Part model, mm, in its own coordinate system. Round coordinates to 2 decimals unless told otherwise and drop trailing zeros. Loops run counter-clockwise (first coordinate to the right, second up) from the corner with the lowest first, then second, coordinate; pieces in that order, holes last.
1) Band-saw the part on D-D, the plane x = 21.5. Write the cut outline in (y, z), then the cut area to 3 significant figures.
2) Band-saw the part on A-A, the plane y = -45. Write the cut outline in (x, z), then the cut area to 3 significant figures.
3) Mould opens along Y. For faces 1 (the flat face through (-1, 1, 2)), 2 (the cylindrical face through (-18, 0, 1)), 3 (the cylindrical face through (23.48, -49.39, 0.99)) say: +Y half, -Y half, draft (parallel to the pull), parting line (faces both ways), or undercut.
4) Band-saw the part on B-B, the plane x = -22.5. Write the cut outline in (y, z), then the cut area to 3 significant figures.
5) Probe line 1 (Y direction, x = -22.5, z = 1.2); line 2 (X direction, y = -41, z = 1.6); line 3 (X direction, y = 47, z = 0.55). List the from-to ranges inside material, lowest first.
6) Band-saw the part on C-C, the plane z = 1.4. Write the cut outline in (x, y).
from build123d import *

# Parameters (mm, degrees)
SKETCH_1_W        = 90
SKETCH_1_H        = 135
EXTRUDE_1_DEPTH   = 2
CHAMFER_1_SIZE    = 2
HOLE_WIZARD_M81_D = 9


with BuildPart() as part:
    # Эскиз1 → Бобышка-Вытянуть1 (new body)
    with BuildSketch(Plane.XY):
        Rectangle(SKETCH_1_W, SKETCH_1_H)
    extrude(amount=EXTRUDE_1_DEPTH)

    # Фаска1
    chamfer_1_edges = [part.edges().sort_by_distance(p)[0] for p in [
        (45, -67.5, 1),
        (-45, -67.5, 1),
        (-45, 67.5, 1),
        (45, 67.5, 1),
    ]]
    chamfer(chamfer_1_edges, length=CHAMFER_1_SIZE)

    # Отверстие с зазором M81 (through all)
    with Locations(Plane.XY.offset(2)):
        with Locations((-22.5, 45), (22.5, 45), (22.5, 0), (-22.5, 0), (-22.5, -45), (22.5, -45)):
            Hole(HOLE_WIZARD_M81_D / 2)


solid = part.part
Reported:
1. outline: (-67.5, 0) - (-49.39, 0) - (-49.39, 2) - (-67.5, 2) - close; (-40.61, 0) - (-4.39, 0) - (-4.39, 2) - (-40.61, 2) - close; (4.39, 0) - (40.61, 0) - (40.61, 2) - (4.39, 2) - close; (49.39, 0) - (67.5, 0) - (67.5, 2) - (49.39, 2) - close
1. area: 217 mm2
2. outline: (-45, 0) - (-27, 0) - (-27, 2) - (-45, 2) - close; (-18, 0) - (18, 0) - (18, 2) - (-18, 2) - close; (27, 0) - (45, 0) - (45, 2) - (27, 2) - close
2. area: 144 mm2
3. face 1: draft
3. face 2: undercut
3. face 3: undercut
4. outline: (-67.5, 0) - (-49.5, 0) - (-49.5, 2) - (-67.5, 2) - close; (-40.5, 0) - (-4.5, 0) - (-4.5, 2) - (-40.5, 2) - close; (4.5, 0) - (40.5, 0) - (40.5, 2) - (4.5, 2) - close; (49.5, 0) - (67.5, 0) - (67.5, 2) - (49.5, 2) - close
4. area: 216 mm2
5. line 1: y = -67.5 to -49.5, -40.5 to -4.5, 4.5 to 40.5, 49.5 to 67.5
5. line 2: x = -45 to -24.56, -20.44 to 20.44, 24.56 to 45
5. line 3: x = -45 to -26.53, -18.47 to 18.47, 26.53 to 45
6. outline: (-45, -65.5) - (-43, -67.5) - (43, -67.5) - (45, -65.5) - (45, 65.5) - (43, 67.5) - (-43, 67.5) - (-45, 65.5) - close; hole circle Ø9 at (-22.5, -45); hole circle Ø9 at (-22.5, 0); hole circle Ø9 at (-22.5, 45); hole circle Ø9 at (22.5, -45); hole circle Ø9 at (22.5, 0); hole circle Ø9 at (22.5, 45)
